Work out the finished part from the listing and answer in its coordinate system (mm). A direction names the side the tool comes from. Coordinates: 2 decimals unless noted, no trailing zeros. Order: outer loops, then holes, each group sorted by start corner. A loop starts at its lowest first (then second) coordinate and runs counter-clockwise, first axis right, second up. Notation, with made-up numbers: M 52.25,65.5 L 64.25,65.5 A26 ccw 64.25,80.5 Z; hole C 85.25,88 d9. An arc over 180 degrees is marked long. Answer in a Markdown table with one row per item. Add a question column.
Item 1: The part is cut by section C-C (z = 21.5). Write down the section's boundary in (x, y).
Item 2: Flat-ended cylindrical pins translate along their axes: pin 1 Ø4 at (x, z) = (-33, 28) entering from +Y; pin 2 Ø8 at (x, z) = (-17, 20) entering from +Y; pin 3 Ø4 at (x, z) = (28, 20.5) entering from -Y. Find the tip coordinate at first contact, or state that the pin passes through.
Item 3: Consider line 1 (Y direction, x = 0, z = 22.5); line 2 (X direction, y = -1.5, z = 24.5); line 3 (X direction, y = 76, z = 20). Determine where each line is inside the solid, lowest interval first. Write a range as from..to.
Item 4: Which of the six approach directions +Z, -Z, +X, -X, +Y, -Y give full straight-line access (tool end or side, diameter ignored) to faces 1 (the face through (75, -52, 30)), 2 (the face through (-16, 103, 0))?
Item 5: The mould has two halves that part along X. Classify faces 3 (the face through (22.106, -99.547, 14.804)), 4 (the face through (78, 48, 31.75)), 5 (the face through (56.985, 89.38, 15.653)): released by +X, released by -X, zero draft, split by the parting line, or undercut.
Item 6: The part is cut by section A-A (y = 0). Write down the section's boundary in (x, z).
from build123d import *

# Parameters (mm, degrees)
BASEPLATE_R         = 106
BASEPLATE_R_2       = 90.414349638
BOSS_EXTRUDE1_DEPTH = 31.75
SKETCH2_R           = 101.971973166
CUT_EXTRUDE1_DEPTH  = 30
FILLET1_R           = 1
FILLET2_R           = 1


with BuildPart() as part:
    # Baseplate → Boss-Extrude1 (new body)
    with BuildSketch(Plane.XY):
        Circle(BASEPLATE_R)
        Circle(BASEPLATE_R_2, mode=Mode.SUBTRACT)
    extrude(amount=BOSS_EXTRUDE1_DEPTH)

    # Sketch2 → Cut-Extrude1 (cut)
    with BuildSketch(Plane(origin=(0, 0, 0), x_dir=(-1, 0, 0), z_dir=(0, 0, -1))):
        Circle(SKETCH2_R)
    extrude(amount=-CUT_EXTRUDE1_DEPTH, mode=Mode.SUBTRACT)

    # Fillet1
    fillet1_edges = [part.edges().sort_by_distance(p)[0] for p in [
        (101.971973166, 0, 0),
    ]]
    fillet(fillet1_edges, radius=FILLET1_R)

    # Fillet2
    fillet2_edges = [part.edges().sort_by_distance(p)[0] for p in [
        (101.971973166, 0, 30),
    ]]
    fillet(fillet2_edges, radius=FILLET2_R)


solid = part.part
Reply:
| question | item | result |
|---|---|---|
| 1 | outline | C 0,0 d212; hole C 0,0 d203.94 |
| 2 | pin 1 | stops at y = 101.37 |
| 2 | pin 2 | stops at y = 105.2 |
| 2 | pin 3 | stops at y = -102.76 |
| 3 | line 1 | y = -106..-101.97, 101.97..106 |
| 3 | line 2 | x = -105.99..-101.96, 101.96..105.99 |
| 3 | line 3 | x = -73.89..-67.99, 67.99..73.89 |
| 4 | face 1 | -Z |
| 4 | face 2 | -Z, +X, -X, +Y, -Y |
| 5 | face 3 | undercut |
| 5 | face 4 | zero draft |
| 5 | face 5 | split by the parting line |
| 6 | outline | M -106,0 L -102.97,0 A1 ccw -101.97,1 L -101.97,29 A1 cw -100.97,30 L -90.41,30 L -90.41,31.75 L -106,31.75 Z; M 90.41,30 L 100.97,30 A1 cw 101.97,29 L 101.97,1 A1 ccw 102.97,0 L 106,0 L 106,31.75 L 90.41,31.75 Z |
